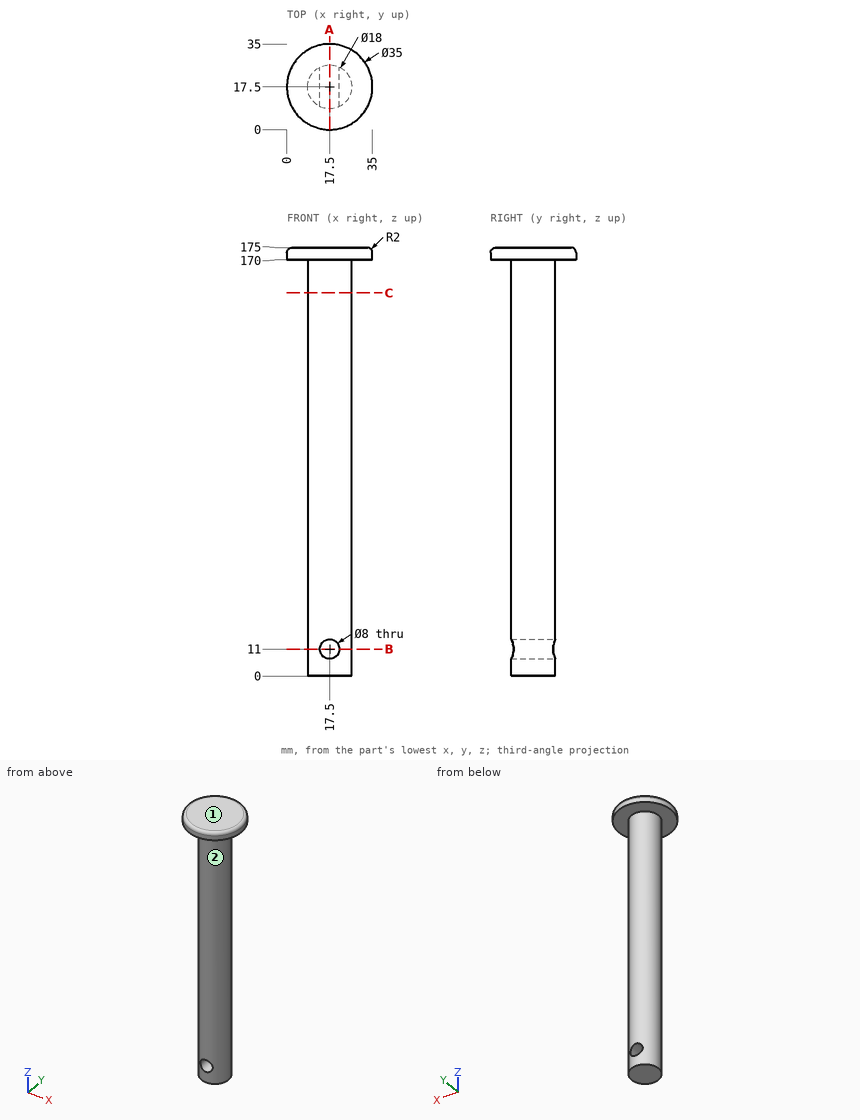
Here's the drawing with two shaded views (mm, measured from the low corner). I have some questions. A direction names the side the tool comes from. Round coordinates to 2 decimals unless told otherwise and drop trailing zeros. Write each loop counter-clockwise with the first axis right and the second up, starting at its lowest first coordinate (ties: lowest second). Pieces come first, ordered by that corner, then holes. Notation, with made-up numbers: M -21,-17 L -7,-17 A29 cw -7,7 Z; hole C 15,19 d7. An arc over 180 degrees is marked long. Use CSV: the item, a comma, the result in double quotes.
(1) Imagine slicing it at C-C (z = 156.5). Write out the boundary of the cut face in (x, y).
Check values:
outline,"C 17.5,17.5 d18"
(2) On a 3-axis mill with a long thin cutter (end or side, diameter ignored), from which of +Z, -Z, +X, -X, +Y, -Y can I reach the whole of each face in a straight line? I mean the marked faces 1 and 2. Say none if no direction works.
Check values:
face 1,"+Z, +X, -X, +Y, -Y"
face 2,"-Z"
(3) I'm going to push flat-ended pins straight in: pin 1 (2 mm diameter, centred on x = 9, z = 28, fed in from -Y); pin 2 (5 mm diameter, centred on y = 26, z = 114, fed in from -X); pin 3 (5 mm diameter, centred on x = 26, z = 31, fed in from -Y). Where does each tip first touch, or does it pass through?
Check values:
pin 1,"y = 12.53"
pin 2,"x = 10.79"
pin 3,"y = 10.79"
(4) Imagine slicing it at A-A (x = 17.5). Write out the boundary of the cut face in (y, z).
Check values:
outline,"M 0,170 L 8.5,170 L 8.5,15 L 26.5,15 L 26.5,170 L 35,170 L 35,173 A2 ccw 33,175 L 2,175 A2 ccw 0,173 Z; M 8.5,0 L 26.5,0 L 26.5,7 L 8.5,7 Z"
(5) Imagine slicing it at B-B (z = 11). Write out the boundary of the cut face in (x, y), plus the area to 3 significant figures.
Check values:
outline,"M 13.5,9.44 L 13.5,25.56 A9 ccw Z; M 21.5,9.44 A9 ccw 21.5,25.56 Z"
area,"115 mm^2"
(6) I need wall thicknesses on line 1 along Z through (x, y) = (17, 18); line 2 along Z through (x, y) = (31, 18); line 3 along Y through (x, z) = (18, 28). Which ranges of each line are inside material? Lowest first, please.
Check values:
line 1,"0 to 7.03, 14.97 to 175"
line 2,"170 to 175"
line 3,"8.51 to 26.49"
